Read the model definition and answer for the solid it produces. Units are mm, in the model's axes. A direction names the side the tool comes from. Coordinates: 2 decimals unless noted, no trailing zeros. Write each loop counter-clockwise with the first axis right and the second up, starting at its lowest first coordinate (ties: lowest second). Pieces come first, ordered by that corner, then holes. Notation, with made-up numbers: M 76.25,83.25 L 126.25,83.25 A24 ccw 126.25,104.25 Z; hole C -21,73 d4. An arc over 180 degrees is marked long. Write item = value, one per line.
from build123d import *

# Parameters (mm, degrees)
F0_W           = 6.35
F0_H           = 142.875
F1_DEPTH       = 38.1
F3_D           = 2.7051
F3_DEPTH       = 15.0876
F3_TIP         = 0.8126940303
F6_D           = 2.2606
F6_DEPTH       = 13.7414
F6_TIP         = 0.6791527577
F6_ON_F4_D     = 2.2606
F6_ON_F4_DEPTH = 13.7414
F6_ON_F4_TIP   = 0.6791527577
F8_DEPTH       = 25.4


with BuildPart() as f1:
    # F0 (on Top) → F1 (new body)
    with BuildSketch(Plane.XY):
        Rectangle(F0_W, F0_H)
    extrude(amount=F1_DEPTH)

    # F3
    with Locations(Plane(origin=(0, 0, 0), x_dir=(1, 0, 0), z_dir=(0, 0, -1))):
        with Locations((0, 46.0375), (0, -46.0375)):
            Hole(F3_D / 2, depth=F3_DEPTH)
            with Locations((0, 0, -(F3_DEPTH + F3_TIP / 2))):  # 118° drill point
                Cone(0, F3_D / 2, F3_TIP, mode=Mode.SUBTRACT)

    # F6
    with Locations(Plane.XZ.offset(71.4375)):
        with Locations((0, 31.75), (0, 6.35)):
            Hole(F6_D / 2, depth=F6_DEPTH)
            with Locations((0, 0, -(F6_DEPTH + F6_TIP / 2))):  # 118° drill point
                Cone(0, F6_D / 2, F6_TIP, mode=Mode.SUBTRACT)

    # F6 on F4
    with Locations(Plane(origin=(0, 71.4375, 0), x_dir=(-1, 0, 0), z_dir=(0, 1, 0))):
        with Locations((0, 25.4), (0, 12.7)):
            Hole(F6_ON_F4_D / 2, depth=F6_ON_F4_DEPTH)
            with Locations((0, 0, -(F6_ON_F4_DEPTH + F6_ON_F4_TIP / 2))):  # 118° drill point
                Cone(0, F6_ON_F4_D / 2, F6_ON_F4_TIP, mode=Mode.SUBTRACT)

    # F7 (on face) → F8 (cut)
    with BuildSketch(Plane(origin=(-3.175, 0, 0), x_dir=(0, -1, 0), z_dir=(-1, 0, 0))):
        with BuildLine():
            Line((-19.4328204888, 26.035), (-40.6460027112, 26.035))
            ThreePointArc((-40.6460027112, 26.035), (-42.7394116, 19.05), (-40.6460027112, 12.065))
            Line((-40.6460027112, 12.065), (-19.4328204888, 12.065))
            ThreePointArc((-19.4328204888, 12.065), (-17.3394116, 19.05), (-19.4328204888, 26.035))
        make_face()
        with BuildLine():
            Line((35.5539972888, 12.065), (56.7671795112, 12.065))
            ThreePointArc((56.7671795112, 12.065), (58.8605884, 19.05), (56.7671795112, 26.035))
            Line((56.7671795112, 26.035), (35.5539972888, 26.035))
            ThreePointArc((35.5539972888, 26.035), (33.4605884, 19.05), (35.5539972888, 12.065))
        make_face()
    extrude(amount=-F8_DEPTH, mode=Mode.SUBTRACT)


solid = f1.part
Item 1: Consider line 1 along Z through (x, y) = (0, -66.5); line 2 along Y through (x, z) = (0, 8.25); line 3 along Y through (x, z) = (0.5, 19.5). Determine where each line is inside the solid, lowest interval first. Write a range as from..to.
Worked answers:
line_1 = 0..5.22, 7.48..30.62, 32.88..38.1
line_2 = -71.44..-47.39, -44.68..44.68, 47.39..71.44
line_3 = -71.44..-58.85, -33.47..17.35, 42.73..71.44
Item 2: Find section A-A (z = 21). Determine the outline of the cut face in (x, y) (1 decimal).
Worked answers:
outline = M -3.2,-71.4 L 3.2,-71.4 L 3.2,-58.7 L -3.2,-58.7 Z; M -3.2,-33.6 L 3.2,-33.6 L 3.2,17.5 L -3.2,17.5 Z; M -3.2,42.6 L 3.2,42.6 L 3.2,71.4 L -3.2,71.4 Z
Item 3: Flat-ended cylindrical pins translate along their axes: pin 1 (2 mm diameter, centred on x = 0, z = 6.35, fed in from -Y); pin 2 (1.4 mm diameter, centred on x = 0, z = 25.4, fed in from +Y). Find the tip coordinate at first contact, or state that the pin passes through.
Worked answers:
pin_1 = -57.62
pin_2 = 57.44
Item 4: Which of the six approach directions +Z, -Z, +X, -X, +Y, -Y give full straight-line access (tool end or side, diameter ignored) to faces 4 (the face through (0.15, -64.47, 7.47)), 5 (the face through (0, 30, 12.065)), 6 (the face through (-0.62, 47.24, 7.65))?
Worked answers:
face_4 = -Y
face_5 = +X, -X
face_6 = -Z
Item 5: For a pull along Z with two mould halves and no side action, classify faces 1 (the face through (-0.15, 64.47, 26.52)), 2 (the face through (-0.727, -47.178, 6.117)), 3 (the face through (0, 1, 0)) as released by +Z, released by -Z, zero draft, split by the parting line, or undercut.
Worked answers:
face_1 = undercut
face_2 = zero draft
face_3 = released by -Z
